The figure shows three views and two pictorial views of one solid part (mm, origin at its lowest corner). Answer the questions. A direction names the side the tool comes from. Give positions to 0.01 mm unless a question says otherwise; leave off trailing zeros. Loops run counter-clockwise (first coordinate to the right, second up) from the corner with the lowest first, then second, coordinate; pieces in that order, holes last. Notation, with made-up numbers: M 64.25,-20 L 104.25,-20 A23 ccw 104.25,-4 Z; hole C 33.5,-25.75 d5. An arc over 180 degrees is marked long. Answer in a Markdown table with one row per item. Add a question column.
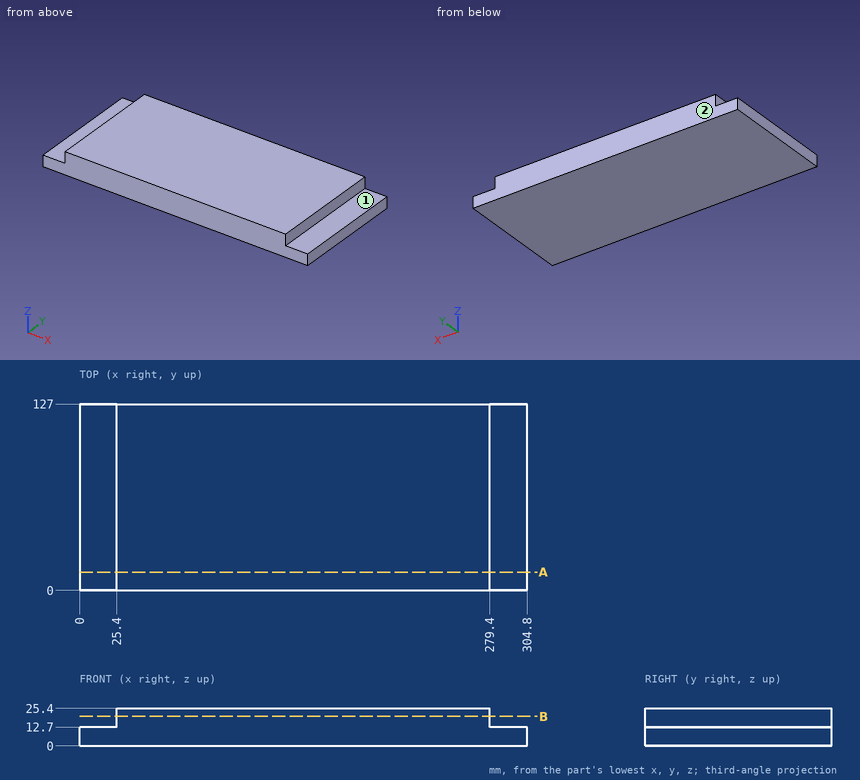
(1) Each of these flat-tipped pins is pushed along its axis until it touches: P1, Ø12, axis at y = 55.5, z = 21, coming from the -X side; P2, Ø12.5, axis at x = 17.5, y = 78, coming from the +Z side. Where does it stop, or does it pass through?
(2) Section B-B, the plane z = 20 is taken. Determine the outline of the cut face in (x, y), and give its area (3 significant figures).
(3) Consider line 1 along X through (y, z) = (61, 20). Determine where the line is inside the solid, lowest interval first. Write a range as from..to.
(4) Section A-A, the plane y = 12.5 is taken. Determine the outline of the cut face in (x, z).
(5) Which of the six approach directions +Z, -Z, +X, -X, +Y, -Y give full straight-line access (tool end or side, diameter ignored) to the marked faces 1 and 2?
Numbers:
| question | item | result |
|---|---|---|
| 1 | P1 | stops at x = 25.4 |
| 1 | P2 | stops at z = 12.7 |
| 2 | outline | M 25.4,0 L 279.4,0 L 279.4,127 L 25.4,127 Z |
| 2 | area | 32,300 mm² |
| 3 | line 1 | x = 25.4..279.4 |
| 4 | outline | M 0,0 L 304.8,0 L 304.8,12.7 L 279.4,12.7 L 279.4,25.4 L 25.4,25.4 L 25.4,12.7 L 0,12.7 Z |
| 5 | face 1 | +Z, +X, +Y, -Y |
| 5 | face 2 | +Z, -Z, +X, -X, +Y |
